The listing builds one solid part. Answer for the finished solid, in the listing's coordinates (mm). A direction names the side the tool comes from. Round coordinates to 2 decimals unless told otherwise and drop trailing zeros. Loops run counter-clockwise (first coordinate to the right, second up) from the corner with the lowest first, then second, coordinate; pieces in that order, holes last. Notation, with made-up numbers: (23, 23) -> (78, 23) arc R20 cw to (78, 45) -> close; hole circle Ø9 at (54.5, 7.25). An arc over 180 degrees is marked (long way). Use a Markdown table: item, result. Add a question column.
Q1. Which of the six approach directions +Z, -Z, +X, -X, +Y, -Y give full straight-line access (tool end or side, diameter ignored) to faces 1 (the cylindrical face through (-19.33, -44.764, 30.302)), 2 (the flat face through (2, 34, -0.25))?
Q2. Given pin 1 Ø2.5 at (x, y) = (-11.12, 55.59) entering from -Z; pin 2 Ø8 at (y, z) = (50.5, 26.5) entering from -X; pin 3 Ø10 at (y, z) = (-51, 3.5) entering from +X; pin 4 Ø6 at (y, z) = (18, -0.5) entering from -X, each flat-ended and moving along its own axis, determine where each tip first touches the part or whether it passes through.
Q3. Section A-A on y = 0 is taken. Give the vertices of the cut face in (x, z) (3 decimals), then the cut area to 3 significant figures.
Q4. Section B-B on x = 101 is taken. Give the vertices of the cut face in (y, z).
Q5. Section C-C on z = 4.5 is taken. Give the vertices of the cut face in (x, y) (1 decimal).
Q6. Consider line 1 (Z direction, x = -16.5, y = 30.5); line 2 (Y direction, x = 34, z = 22); line 3 (X direction, y = -6, z = 0.5). Determine where each line is inside the solid, lowest interval first.
Q7. For a pull along X with two mould halves and no side action, classify faces 3 (the cylindrical face through (92.647, 46.935, -2.828)), 4 (the flat face through (69, 16, -4.06)), 5 (the cylindrical face through (-10.246, 53.909, 30.302)), 6 (the cylindrical face through (71.31, 69.33, -2.18)) as released by +X, released by -X, zero draft, split by the parting line, or undercut.
from build123d import *

# Parameters (mm, degrees)
SKETCH2_R          = 1.8288
CUT_EXTRUDE1_DEPTH = 143.234851149
CIRPATTERN1_COUNT  = 4


# Read off the part's stored shape, not the designer's step: CSK for #6 Flat Head Machine Screw (100)1
with BuildPart() as part:
    # Sketch1 → Revolve8 (revolve)
    with BuildSketch(Plane(origin=(0, 0, 0), x_dir=(1, 0, 0), z_dir=(0, 1, 0)), mode=Mode.PRIVATE) as revolve8_sk:
        with BuildLine():
            Line((-42.91, 4.059999872), (-1, 4.059999872))
            Line((-1, 4.059999872), (-1, -31.500000128))
            Line((-1, -31.500000128), (-42.91, -31.500000128))
            Line((-42.91, -31.500000128), (-42.91, -27.690000128))
            Line((-42.91, -27.690000128), (-6.08, -27.690000128))
            ThreePointArc((-6.08, -27.690000128), (-5.181974388, -27.31802574), (-4.81, -26.420000128))
            Line((-4.81, -26.420000128), (-4.81, -1.020000128))
            ThreePointArc((-4.81, -1.020000128), (-5.181974388, -0.121974516), (-6.08, 0.249999872))
            Line((-6.08, 0.249999872), (-42.91, 0.249999872))
            Line((-42.91, 0.249999872), (-42.91, 4.059999872))
        make_face()
    revolve(revolve8_sk.sketch.rotate(Axis((35.2425, 0, 32.45), (0, 0, -1)), 180), axis=Axis((35.2425, 0, 32.45), (0, 0, -1)))

    # Sketch2 → Cut-Extrude1 (cut, through all)
    with BuildSketch(Plane(origin=(0, 0, -4.059999872), x_dir=(-1, 0, 0), z_dir=(0, 0, -1))):
        with Locations((11.122317884, 55.593306815)):
            Circle(SKETCH2_R)
    cut_extrude1 = extrude(amount=-CUT_EXTRUDE1_DEPTH, mode=Mode.SUBTRACT)

    # CirPattern1: Cut-Extrude1 ×4 about axis
    cirpattern1_axis = Axis((35.2425, 0, 0), (0, 0, 1))
    for i in range(1, CIRPATTERN1_COUNT):
        add(cut_extrude1.rotate(cirpattern1_axis, i * 360 / CIRPATTERN1_COUNT), mode=Mode.SUBTRACT)

    # CSK for _6 Flat Head Machine Screw _ 2 → CSK for #6 Flat Head Machine Screw (100)1 (revolve, cut)
    with BuildSketch(Plane(origin=(-11.122317884, 55.593306815, 0), x_dir=(1, 0, 0), z_dir=(0, -1, 0))):
        Polygon((1.89865, 29.070025336), (1.89865, 31.500000128), (1.8288, 31.500000128), (1.8288, 27.690000128), (3.5433, 27.690000128), align=None)
        Polygon((1.89865, -1.63002508), (3.5433, -0.249999872), (1.8288, -0.249999872), (1.8288, -4.059999872), (1.89865, -4.059999872), align=None)
    revolve(axis=Axis((-11.122317884, 55.593306815, 0), (0, 0, 1)), mode=Mode.SUBTRACT)

    # CSK for _6 Flat Head Machine Screw _ 3 o → CSK for _6 Flat Head Machine Screw _ 3 (revolve, cut)
    with BuildSketch(Plane(origin=(-20.350806815, -46.364817884, 0), x_dir=(1, 0, 0), z_dir=(0, -1, 0))):
        Polygon((1.89865, 29.070025336), (1.89865, 31.500000128), (1.8288, 31.500000128), (1.8288, 27.690000128), (3.5433, 27.690000128), align=None)
        Polygon((1.89865, -1.63002508), (3.5433, -0.249999872), (1.8288, -0.249999872), (1.8288, -4.059999872), (1.89865, -4.059999872), align=None)
    revolve(axis=Axis((-20.350806815, -46.364817884, 0), (0, 0, 1)), mode=Mode.SUBTRACT)

    # CSK for _6 Flat Head Machine Screw _ 4 o → CSK for _6 Flat Head Machine Screw _ 4 (revolve, cut)
    with BuildSketch(Plane(origin=(81.607317884, -55.593306815, 0), x_dir=(1, 0, 0), z_dir=(0, -1, 0))):
        Polygon((1.89865, 29.070025336), (1.89865, 31.500000128), (1.8288, 31.500000128), (1.8288, 27.690000128), (3.5433, 27.690000128), align=None)
        Polygon((1.89865, -1.63002508), (3.5433, -0.249999872), (1.8288, -0.249999872), (1.8288, -4.059999872), (1.89865, -4.059999872), align=None)
    revolve(axis=Axis((81.607317884, -55.593306815, 0), (0, 0, 1)), mode=Mode.SUBTRACT)

    # CSK for _6 Flat Head Machine Screw _ 5 o → CSK for _6 Flat Head Machine Screw _ 5 (revolve, cut)
    with BuildSketch(Plane(origin=(90.835806815, 46.364817884, 0), x_dir=(1, 0, 0), z_dir=(0, -1, 0))):
        Polygon((1.89865, 29.070025336), (1.89865, 31.500000128), (1.8288, 31.500000128), (1.8288, 27.690000128), (3.5433, 27.690000128), align=None)
        Polygon((1.89865, -1.63002508), (3.5433, -0.249999872), (1.8288, -0.249999872), (1.8288, -4.059999872), (1.89865, -4.059999872), align=None)
    revolve(axis=Axis((90.835806815, 46.364817884, 0), (0, 0, 1)), mode=Mode.SUBTRACT)


solid = part.part
Checked values:
| question | item | result |
|---|---|---|
| 1 | face 1 | +Z, -Z |
| 1 | face 2 | none |
| 2 | pin 1 | passes through |
| 2 | pin 2 | stops at x = -27.44 |
| 2 | pin 3 | stops at x = 97.16 |
| 2 | pin 4 | stops at x = -41.46 |
| 3 | outline | (-42.91, -4.06) -> (-1, -4.06) -> (-1, 31.5) -> (-42.91, 31.5) -> (-42.91, 27.69) -> (-6.08, 27.69) arc R1.27 cw to (-4.81, 26.42) -> (-4.81, 1.02) arc R1.27 cw to (-6.08, -0.25) -> (-42.91, -0.25) -> close; (71.485, -4.06) -> (113.395, -4.06) -> (113.395, -0.25) -> (76.565, -0.25) arc R1.27 cw to (75.295, 1.02) -> (75.295, 26.42) arc R1.27 cw to (76.565, 27.69) -> (113.395, 27.69) -> (113.395, 31.5) -> (71.485, 31.5) -> close |
| 3 | area | 853 mm2 |
| 4 | outline | (-42.23, -4.06) -> (42.23, -4.06) -> (42.23, -0.25) -> (-42.23, -0.25) -> close; (-42.23, 27.69) -> (42.23, 27.69) -> (42.23, 31.5) -> (-42.23, 31.5) -> close |
| 5 | outline | circle Ø80.1 at (35.2, 0); hole circle Ø72.5 at (35.2, 0) |
| 6 | line 1 | z = -4.06 to -0.25, 27.69 to 31.5 |
| 6 | line 2 | y = -40.03 to -36.22, 36.22 to 40.03 |
| 6 | line 3 | x = -4.47 to -0.5, 70.98 to 74.96 |
| 7 | face 3 | undercut |
| 7 | face 4 | zero draft |
| 7 | face 5 | undercut |
| 7 | face 6 | split by the parting line |
